from build123d import *

# Parameters (mm, degrees)
BOSS_EXTRUDE3_DEPTH = 10
FILLET3_R           = 10
SKETCH2_R           = 2.5
CUT_EXTRUDE1_DEPTH  = 100
SKETCH3_R           = 2.5
CUT_EXTRUDE3_DEPTH  = 100
SKETCH4_R           = 5
CUT_EXTRUDE4_DEPTH  = 5
SKETCH5_R           = 2.25
CUT_EXTRUDE7_DEPTH  = 5
SKETCH8_R           = 2.25
CUT_EXTRUDE8_DEPTH  = 5
SKETCH9_R           = 2.25
CUT_EXTRUDE9_DEPTH  = 5
SKETCH10_R          = 5
CUT_EXTRUDE13_DEPTH = 12
SKETCH12_R          = 2.5
CUT_EXTRUDE14_DEPTH = 12


with BuildPart() as part:
    # Sketch1 → Boss-Extrude3 (new body)
    with BuildSketch(Plane(origin=(0, 0, 0), x_dir=(1, 0, 0), z_dir=(0, 1, 0))):
        Polygon((60, 150), (60, 160), (0, 160), (0, 80), (45, 80), (45, 150), align=None)
        Polygon((120, 160), (60, 160), (60, 150), (75, 150), (75, 80), (120, 80), align=None)
        Polygon((120, 0), (120, 80), (75, 80), (75, 20), (60, 20), (60, 0), align=None)
        Polygon((45, 80), (0, 80), (0, 0), (60, 0), (60, 20), (45, 20), align=None)
    extrude(amount=BOSS_EXTRUDE3_DEPTH)

    # Fillet3
    fillet3_edges = [part.edges().sort_by_distance(p)[0] for p in [
        (75, 5, -150),
        (45, 5, -150),
        (45, 5, -20),
        (75, 5, -20),
    ]]
    fillet(fillet3_edges, radius=FILLET3_R)

    # Sketch2 → Cut-Extrude1 (cut)
    with BuildSketch(Plane(origin=(0, 10, 0), x_dir=(1, 0, 0), z_dir=(0, 1, 0))):
        with Locations(Location((19, 153.5, 0), (0, 0, 270))):
            Circle(SKETCH2_R)
        with Locations(Location((6.5, 141, 0), (0, 0, 270))):
            Circle(SKETCH2_R)
    extrude(amount=-CUT_EXTRUDE1_DEPTH, mode=Mode.SUBTRACT)

    # Sketch3 → Cut-Extrude3 (cut)
    with BuildSketch(Plane(origin=(0, 10, 0), x_dir=(1, 0, 0), z_dir=(0, 1, 0))):
        with Locations(Location((113.5, 141, 0), (0, 0, 270))):
            Circle(SKETCH3_R)
        with Locations(Location((101, 153.5, 0), (0, 0, 270))):
            Circle(SKETCH3_R)
    extrude(amount=-CUT_EXTRUDE3_DEPTH, mode=Mode.SUBTRACT)

    # Sketch4 → Cut-Extrude4 (cut)
    with BuildSketch(Plane.XZ):
        with Locations(Location((113.5, -141, 0), (0, 0, 270))):
            Circle(SKETCH4_R)
        with Locations(Location((101, -153.5, 0), (0, 0, 270))):
            Circle(SKETCH4_R)
        with Locations(Location((19, -153.5, 0), (0, 0, 270))):
            Circle(SKETCH4_R)
        with Locations(Location((6.5, -141, 0), (0, 0, 270))):
            Circle(SKETCH4_R)
    extrude(amount=-CUT_EXTRUDE4_DEPTH, mode=Mode.SUBTRACT)

    # Sketch5 → Cut-Extrude7 (cut)
    with BuildSketch(Plane.XZ):
        with Locations(Location((112.5, -152.5, 0), (0, 0, 270))):
            Circle(SKETCH5_R)
    extrude(amount=-CUT_EXTRUDE7_DEPTH, mode=Mode.SUBTRACT)

    # Sketch8 → Cut-Extrude8 (cut)
    with BuildSketch(Plane(origin=(0, 0, 0), x_dir=(-1, 0, 0), z_dir=(0, -1, 0))):
        with Locations(Location((-7.5, 153.623044918, 0), (0, 0, 90))):
            Circle(SKETCH8_R)
    extrude(amount=-CUT_EXTRUDE8_DEPTH, mode=Mode.SUBTRACT)

    # Sketch9 → Cut-Extrude9 (cut)
    with BuildSketch(Plane(origin=(0, 0, 0), x_dir=(-1, 0, 0), z_dir=(0, -1, 0))):
        with Locations(Location((-7.5, 7.5, 0), (0, 0, 90))):
            Circle(SKETCH9_R)
        with Locations(Location((-112.5, 7.5, 0), (0, 0, 90))):
            Circle(SKETCH9_R)
    extrude(amount=-CUT_EXTRUDE9_DEPTH, mode=Mode.SUBTRACT)

    # Sketch10 → Cut-Extrude13 (cut)
    with BuildSketch(Plane(origin=(0, 5, 0), x_dir=(-1, 0, 0), z_dir=(0, -1, 0))):
        with Locations(Location((-80, 7.5, 0), (0, 0, 270))):
            Circle(SKETCH10_R)
        with Locations(Location((-40, 7.5, 0), (0, 0, 270))):
            Circle(SKETCH10_R)
    extrude(amount=CUT_EXTRUDE13_DEPTH, mode=Mode.SUBTRACT)

    # Sketch12 → Cut-Extrude14 (cut)
    with BuildSketch(Plane(origin=(0, 5, 0), x_dir=(-1, 0, 0), z_dir=(0, -1, 0))):
        with Locations(Location((-80, 7.5, 0), (0, 0, 90))):
            Circle(SKETCH12_R)
        with Locations(Location((-40, 7.5, 0), (0, 0, 90))):
            Circle(SKETCH12_R)
    extrude(amount=-CUT_EXTRUDE14_DEPTH, mode=Mode.SUBTRACT)


solid = part.part
The listing builds one solid part. Answer for the finished solid, in the listing's coordinates (mm). A direction names the side the tool comes from. Round coordinates to 2 decimals unless told otherwise and drop trailing zeros. Order: outer loops, then holes, each group sorted by start corner. A loop starts at its lowest first (then second) coordinate and runs counter-clockwise, first axis right, second up. Notation, with made-up numbers: (28.5, -20.5) -> (32.5, -20.5) arc R14 ccw to (32.5, -15.5) -> close; hole circle Ø2 at (40, -26). An arc over 180 degrees is marked (long way). Put each result on its own line as item: value.
Q1. This flat-tipped pin is pushed along its axis until it touches: P1, Ø8, axis at x = 101, z = -153.5, coming from the -Y side. Where does it stop, or does it pass through?
Results list:
P1: y = 5
Q2. Determine the mould class of faces 4 (the flat face through (60, 5, -150)), 5 (the flat face through (59, 5, 0)), 6 (the flat face through (0, 5, -81)) for opening direction X: pulls with the +X half, pulls with the -X half, needs draft (parallel to the pull), parting line crosses it, or undercut.
Results list:
face 4: undercut
face 5: needs draft
face 6: pulls with the -X half
Q3. Section D-D, the plane z = -68 is taken. Write down the section's boundary in (x, y).
Results list:
outline: (0, 0) -> (45, 0) -> (45, 10) -> (0, 10) -> close; (75, 0) -> (120, 0) -> (120, 10) -> (75, 10) -> close
Q4. Section B-B, the plane x = 47 is taken. Write down the section's boundary in (y, z).
Results list:
outline: (0, -160) -> (10, -160) -> (10, -146) -> (0, -146) -> close; (0, -24) -> (10, -24) -> (10, 0) -> (0, 0) -> close
Q5. Section C-C, the plane y = 8 is taken. Write down the section's boundary in (x, z).
Results list:
outline: (0, -160) -> (120, -160) -> (120, 0) -> (0, 0) -> close; hole circle Ø5 at (6.5, -141); hole circle Ø5 at (19, -153.5); hole circle Ø5 at (40, -7.5); hole (45, -140) arc R10 ccw to (55, -150) -> (65, -150) arc R10 ccw to (75, -140) -> (75, -30) arc R10 ccw to (65, -20) -> (55, -20) arc R10 ccw to (45, -30) -> close; hole circle Ø5 at (80, -7.5); hole circle Ø5 at (101, -153.5); hole circle Ø5 at (113.5, -141)
Q6. Section A-A, the plane z = -7.5 is taken. Write down the section's boundary in (x, y).
Results list:
outline: (0, 0) -> (5.25, 0) -> (5.25, 5) -> (9.75, 5) -> (9.75, 0) -> (35, 0) -> (35, 5) -> (37.5, 5) -> (37.5, 10) -> (0, 10) -> close; (42.5, 5) -> (45, 5) -> (45, 0) -> (75, 0) -> (75, 5) -> (77.5, 5) -> (77.5, 10) -> (42.5, 10) -> close; (82.5, 5) -> (85, 5) -> (85, 0) -> (110.25, 0) -> (110.25, 5) -> (114.75, 5) -> (114.75, 0) -> (120, 0) -> (120, 10) -> (82.5, 10) -> close
Q7. Consider line 1 along X through (y, z) = (6.15, -7.5); line 2 along X through (y, z) = (6.4, -153.5); line 3 along X through (y, z) = (3.8, -141). Determine where each line is inside the solid, lowest interval first.
Results list:
line 1: 0 to 37.5, 42.5 to 77.5, 82.5 to 120
line 2: 0 to 16.5, 21.5 to 98.5, 103.5 to 120
line 3: 0 to 1.5, 11.5 to 45.05, 74.95 to 108.5, 118.5 to 120
Q8. Which of the six approach directions +Z, -Z, +X, -X, +Y, -Y give full straight-line access (tool end or side, diameter ignored) to faces 1 (the cylindrical face through (101.22, 2.465, -148.505)), 2 (the flat face through (32, 0, -81)), 3 (the cylindrical face through (48.01, 5.07, -147.15))?
Results list:
face 1: -Y
face 2: +Z, -Z, +X, -X, -Y
face 3: +Y, -Y
